from build123d import *

# Parameters (mm, degrees)
F0_W      = 68.5
F0_H      = 25
F1_DEPTH  = 1
F2_W      = 68.5
F2_H      = 1
F3_DEPTH  = 23
F4_W      = 1
F4_H      = 24
F5_DEPTH  = 23
F6_W      = 67.5
F6_H      = 1
F7_DEPTH  = 23
F8_W      = 6
F8_H      = 4.5
F9_DEPTH  = 1
F10_W     = 22.405751
F10_H     = 22.382014
F11_DEPTH = 25


with BuildPart() as f1:
    # F0 (on Front) → F1 (new body)
    with BuildSketch(Plane.XZ):
        Rectangle(F0_W, F0_H)
    extrude(amount=F1_DEPTH)

    # F2 (on face) → F3 (join)
    with BuildSketch(Plane(origin=(0, 0, 0), x_dir=(-1, 0, 0), z_dir=(0, 1, 0))):
        with Locations((0, -12)):
            Rectangle(F2_W, F2_H)
    extrude(amount=F3_DEPTH)

    # F4 (on face) → F5 (join)
    with BuildSketch(Plane(origin=(0, 0, 0), x_dir=(-1, 0, 0), z_dir=(0, 1, 0))):
        with Locations((-33.75, 0.5)):
            Rectangle(F4_W, F4_H)
    extrude(amount=F5_DEPTH)

    # F6 (on face) → F7 (join)
    with BuildSketch(Plane(origin=(0, 0, 0), x_dir=(-1, 0, 0), z_dir=(0, 1, 0))):
        with Locations((0.5, 12)):
            Rectangle(F6_W, F6_H)
    extrude(amount=F7_DEPTH)

    # F8 (on face) → F9 (cut, through all)
    with BuildSketch(Plane.YZ.offset(34.25)):
        with Locations((11, 0)):
            Rectangle(F8_W, F8_H)
    extrude(amount=-F9_DEPTH, mode=Mode.SUBTRACT)

    # F10 (on face) → F11 (cut)
    with BuildSketch(Plane(origin=(0, 0, -12.5), x_dir=(1, 0, 0), z_dir=(0, 0, -1))):
        with Locations((20.026559, -11.808993)):
            Rectangle(F10_W, F10_H)
    extrude(amount=-F11_DEPTH, mode=Mode.SUBTRACT)


solid = f1.part
Here's how the part is built. I have some questions about the finished solid (model axes, mm). A direction names the side the tool comes from. Coordinates: 2 decimals unless noted, no trailing zeros. Order: outer loops, then holes, each group sorted by start corner. A loop starts at its lowest first (then second) coordinate and runs counter-clockwise, first axis right, second up.
Item 1: For P1, Ø11.5, axis at x = -0.5, z = -2, coming from the +Y side; P2, Ø11.5, axis at x = 15, y = 7.5, coming from the -Z side; P3, Ø11.5, axis at y = 15, z = -0.5, coming from the -X side; P4, Ø0.8, axis at x = 21, z = 12, coming from the +Y side, each with a flat end and sliding along its axis, tell me the tip position at first contact or that it passes through.
Result sheet:
P1: stops at y = 0
P2: passes through
P3: stops at x = 33.25
P4: stops at y = 0.62
Item 2: I need wall thicknesses on line 1 (Z direction, x = -29.5, y = 2.75); line 2 (Y direction, x = 13.5, z = -2); line 3 (X direction, y = 3.75, z = -7.5). Which ranges of each line are inside material? Lowest first, please.
Result sheet:
line 1: z = -12.5 to -11.5, 11.5 to 12.5
line 2: y = -1 to 0
line 3: x = 33.25 to 34.25
Item 3: For faces 5 (the face through (34.25, 11, -3)), 6 (the face through (-15, 11, -11.5)), which set-ups out of +Z, -Z, +X, -X, +Y, -Y let a thin tool reach every point of the face, with its end or its side?
Result sheet:
face 5: +Z, -Z, +X, +Y, -Y
face 6: -X, +Y
Item 4: If we section it at C-C on y = 13: List the corners of the cut face in (x, z) for me.
Result sheet:
outline: (-34.25, -12.5) - (8.82, -12.5) - (8.82, -11.5) - (-34.25, -11.5) - close; (-34.25, 11.5) - (8.82, 11.5) - (8.82, 12.5) - (-34.25, 12.5) - close; (31.23, -12.5) - (34.25, -12.5) - (34.25, -2.25) - (33.25, -2.25) - (33.25, -11.5) - (31.23, -11.5) - close; (31.23, 11.5) - (33.25, 11.5) - (33.25, 2.25) - (34.25, 2.25) - (34.25, 12.5) - (31.23, 12.5) - close
Item 5: If we section it at A-A on z = 1.25: List the corners of the cut face in (x, y) for me, plus the area to 3 significant figures.
Result sheet:
outline: (-34.25, -1) - (34.25, -1) - (34.25, 8) - (33.25, 8) - (33.25, 0) - (-34.25, 0) - close; (33.25, 14) - (34.25, 14) - (34.25, 23) - (33.25, 23) - close
area: 85.5 mm2
Item 6: If we mould it in two halves opening along Z, with no side actions, what happens to faces 1 (the face through (0, -1, 0)), 2 (the face through (-1, 0, 0)), 3 (the face through (-15, 11, 11.5)), 4 (the face through (-7, 11, 12.5))? For each: +Z half, -Z half, draft (parallel to the pull), parting line (faces both ways), or undercut.
Result sheet:
face 1: draft
face 2: undercut
face 3: undercut
face 4: +Z half
Item 7: If we section it at D-D on x = -6: List the corners of the cut face in (y, z) for me.
Result sheet:
outline: (-1, -12.5) - (23, -12.5) - (23, -11.5) - (0, -11.5) - (0, 11.5) - (23, 11.5) - (23, 12.5) - (-1, 12.5) - close
Item 8: If we section it at B-B on y = 20.25: List the corners of the cut face in (x, z) for me.
Result sheet:
outline: (-34.25, -12.5) - (8.82, -12.5) - (8.82, -11.5) - (-34.25, -11.5) - close; (-34.25, 11.5) - (8.82, 11.5) - (8.82, 12.5) - (-34.25, 12.5) - close; (31.23, -12.5) - (34.25, -12.5) - (34.25, 12.5) - (31.23, 12.5) - (31.23, 11.5) - (33.25, 11.5) - (33.25, -11.5) - (31.23, -11.5) - close
